from build123d import *

# Parameters (mm, degrees)
SKETCH1_W                   = 20
SKETCH1_H                   = 5
BOSS_EXTRUDE1_DEPTH         = 100
M3_TAPPED_HOLE2_D           = 2.5
M3_TAPPED_HOLE2_CSINK_D     = 3.05
M3_TAPPED_HOLE2_CSINK_ANGLE = 90
LPATTERN1_COUNT             = 2
LPATTERN1_PITCH             = 70


with BuildPart() as part:
    # Sketch1 → Boss-Extrude1 (new body)
    with BuildSketch(Plane.XY):
        Rectangle(SKETCH1_W, SKETCH1_H)
    extrude(amount=BOSS_EXTRUDE1_DEPTH)

    # M3 Tapped Hole2 (through all)
    with Locations(Plane(origin=(0, 2.5, 0), x_dir=(1, 0, 0), z_dir=(0, 1, 0))):
        with Locations((4.698821008, -14.236441586)):
            m3_tapped_hole2 = CounterSinkHole(M3_TAPPED_HOLE2_D / 2, M3_TAPPED_HOLE2_CSINK_D / 2, counter_sink_angle=M3_TAPPED_HOLE2_CSINK_ANGLE)

    # LPattern1: M3 Tapped Hole2 ×2
    with Locations(*[(0, 0, i * LPATTERN1_PITCH) for i in range(1, LPATTERN1_COUNT)]):
        add(m3_tapped_hole2, mode=Mode.SUBTRACT)


solid = part.part
Source: CAD feature listing. Evaluate the final solid. Frame: model axes, mm. Coordinates: 2 decimals unless noted, no trailing zeros. Write each question's results on one line, items separated by ' | '. Start each with the question number.
Item 1: First-contact query: pin 1 Ø3 at (x, y) = (5.5, 1.5) entering from -Z. Flat tip, straight axial feed; report the tip coordinate or a pass-through.
Item 2: Line query: probe 1 along Z at (x, y) = (4.75, 0.65); probe 2 along X at (y, z) = (-1.75, 15); probe 3 along Z at (x, y) = (4, 2). Output: solid intervals per line, ascending.
Item 3: Draft query along X for faces 1 (the face through (4, -0.2, 83.2)), 2 (the face through (-10, 0, 49)), 3 (the face through (0, -2.5, 49)), 4 (the face through (10, 0, 49)). Return one class per face: pulls with the +X half, pulls with the -X half, needs draft (parallel to the pull), parting line crosses it, or undercut.
Checked values:
1) pin 1: stops at z = 0
2) probe 1: z = 0 to 12.99, 15.49 to 82.99, 85.49 to 100 | probe 2: x = -10 to 3.71, 5.69 to 10 | probe 3: z = 0 to 13.2, 15.27 to 83.2, 85.27 to 100
3) face 1: undercut | face 2: pulls with the -X half | face 3: needs draft | face 4: pulls with the +X half
